For this review, take the finished solid that the model builds, in its own axes (mm). A direction names the side the tool comes from. Give positions to 0.01 mm unless a question says otherwise; leave off trailing zeros. Write each loop counter-clockwise with the first axis right and the second up, starting at its lowest first coordinate (ties: lowest second). Pieces come first, ordered by that corner, then holes.
from build123d import *

# Parameters (mm, degrees)
SKETCH1_W                = 79.7
SKETCH1_H                = 100
SKETCH1_R                = 3.5
SKETCH1_W_2              = 10.2
SKETCH1_H_2              = 10.2
SKETCH1_W_3              = 11
SKETCH1_H_3              = 3
SKETCH1_W_4              = 3
BOSS_EXTRUDE1_DEPTH      = 2
BOSS_EXTRUDE2_DEPTH      = 2
BOSS_EXTRUDE2_DEPTH_BACK = 10
SKETCH1_3_W              = 83.7
SKETCH1_3_H              = 104
SKETCH1_3_W_2            = 79.7
SKETCH1_3_H_2            = 100


with BuildPart() as part:
    # Sketch1 → Boss-Extrude1 (new body)
    with BuildSketch(Plane(origin=(0, 0, 0), x_dir=(1, 0, 0), z_dir=(0, 1, 0))):
        with Locations((-77.999694214, 27.678571429)):
            Rectangle(SKETCH1_W, SKETCH1_H)
        with Locations(Location((-102.849694214, 35.042631833, 0), (0, 0, 270))):
            Circle(SKETCH1_R, mode=Mode.SUBTRACT)
        with Locations(Location((-86.349694214, 35.042631833, 0), (0, 0, 270))):
            Circle(SKETCH1_R, mode=Mode.SUBTRACT)
        with Locations(Location((-69.849694214, 35.042631833, 0), (0, 0, 270))):
            Circle(SKETCH1_R, mode=Mode.SUBTRACT)
        with Locations(Location((-53.349694214, 35.042631833, 0), (0, 0, 270))):
            Circle(SKETCH1_R, mode=Mode.SUBTRACT)
        with Locations(Location((-102.849694214, 50.042631833, 0), (0, 0, 270))):
            Circle(SKETCH1_R, mode=Mode.SUBTRACT)
        with Locations(Location((-86.349694214, 50.042631833, 0), (0, 0, 270))):
            Circle(SKETCH1_R, mode=Mode.SUBTRACT)
        with Locations(Location((-69.849694214, 50.042631833, 0), (0, 0, 270))):
            Circle(SKETCH1_R, mode=Mode.SUBTRACT)
        with Locations(Location((-53.349694214, 50.042631833, 0), (0, 0, 270))):
            Circle(SKETCH1_R, mode=Mode.SUBTRACT)
        with Locations((-86.249694214, -10.078571429)):
            Rectangle(SKETCH1_W_2, SKETCH1_H_2, mode=Mode.SUBTRACT)
        with Locations((-102.749694214, -10.078571429)):
            Rectangle(SKETCH1_W_2, SKETCH1_H_2, mode=Mode.SUBTRACT)
        with Locations((-69.749694214, -10.078571429)):
            Rectangle(SKETCH1_W_2, SKETCH1_H_2, mode=Mode.SUBTRACT)
        with Locations((-53.249694214, -10.078571429)):
            Rectangle(SKETCH1_W_2, SKETCH1_H_2, mode=Mode.SUBTRACT)
        with Locations((-86.249694214, 14.921428571)):
            Rectangle(SKETCH1_W_2, SKETCH1_H_2, mode=Mode.SUBTRACT)
        with Locations((-102.749694214, 14.921428571)):
            Rectangle(SKETCH1_W_2, SKETCH1_H_2, mode=Mode.SUBTRACT)
        with Locations((-69.749694214, 14.921428571)):
            Rectangle(SKETCH1_W_2, SKETCH1_H_2, mode=Mode.SUBTRACT)
        with Locations((-53.249694214, 14.921428571)):
            Rectangle(SKETCH1_W_2, SKETCH1_H_2, mode=Mode.SUBTRACT)
        with Locations((-78.657921682, 69.115214956)):
            Rectangle(SKETCH1_W_3, SKETCH1_H_3, mode=Mode.SUBTRACT)
        with Locations((-112.817389032, 69.702349137)):
            Rectangle(SKETCH1_W_4, SKETCH1_H_2, mode=Mode.SUBTRACT)
        with Locations((-105.072966437, 69.702349137)):
            Rectangle(SKETCH1_W_2, SKETCH1_H_2, mode=Mode.SUBTRACT)
    extrude(amount=BOSS_EXTRUDE1_DEPTH)

    # Sketch1<3> → Boss-Extrude2 (add, two sides: drawn at the far end of the back side and taken through both)
    with BuildSketch(Plane(origin=(0, 0, 0), x_dir=(1, 0, 0), z_dir=(0, 1, 0)).offset(-BOSS_EXTRUDE2_DEPTH_BACK)):
        with Locations((-77.999694214, 27.678571429)):
            Rectangle(SKETCH1_3_W, SKETCH1_3_H)
        with Locations((-77.999694214, 27.678571429)):
            Rectangle(SKETCH1_3_W_2, SKETCH1_3_H_2, mode=Mode.SUBTRACT)
    extrude(amount=BOSS_EXTRUDE2_DEPTH + BOSS_EXTRUDE2_DEPTH_BACK)


solid = part.part
(1) For L1, parallel to Z at x = -53, y = -8.5; L2, parallel to X at y = -0.5, z = -65.5; L3, parallel to Z at x = -81.5, y = 0.75, list the stretches that pass through material, from the lowest coordinate up.
(2) We need section C-C (z = -72). Write out the cut boundary in (x, y), and give its area (3 significant figures).
(3) We need section B-B (y = -1.25). Write out the cut boundary in (x, z).
(4) We need section D-D (x = -92.5). Write out the cut boundary in (y, z), and give its area (3 significant figures).
(5) The part is to be moulded in two halves that separate along X. For faces 3 (the cylindrical face through (-50.98, 0.99, -37.62)), 4 (the flat face through (-36.15, -4, -27)), 5 (the flat face through (-119.85, -4, -27)), 6 (the flat face through (-79, -4, 24.321)), say which applies: +X half, -X half, draft (parallel to the pull), parting line (faces both ways), or undercut.
(6) Tool access review of faces 1 (the flat face through (-79, 0, -28)), 2 (the flat face through (-78, -10, -78)): name each direction out of +Z, -Z, +X, -X, +Y, -Y from which nothing blocks a thin tool from reaching the whole face with its end or side.
(7) Clearance check with a flat-ended pin moving along its axis: pin 1 Ø1.5 at (x, z) = (-49.5, -25) entering from -Y. State where the tip first meets the part, or that it passes through.
(8) We need section A-A (z = 7). Write out the cut boundary in (x, y).
The answers:
1. L1: z = -79.68 to -77.68, 22.32 to 24.32
1. L2: x = -119.85 to -117.85, -38.15 to -36.15
1. L3: z = -79.68 to -70.62, -67.62 to -20.02, -9.82 to 4.98, 15.18 to 24.32
2. outline: (-119.85, -10) - (-117.85, -10) - (-117.85, 0) - (-114.32, 0) - (-114.32, 2) - (-119.85, 2) - close; (-111.32, 0) - (-110.17, 0) - (-110.17, 2) - (-111.32, 2) - close; (-99.97, 0) - (-38.15, 0) - (-38.15, -10) - (-36.15, -10) - (-36.15, 2) - (-99.97, 2) - close
2. area: 181 mm2
3. outline: (-119.85, -79.68) - (-36.15, -79.68) - (-36.15, 24.32) - (-119.85, 24.32) - close; hole (-117.85, -77.68) - (-38.15, -77.68) - (-38.15, 22.32) - (-117.85, 22.32) - close
4. outline: (-10, -79.68) - (2, -79.68) - (2, 24.32) - (-10, 24.32) - (-10, 22.32) - (0, 22.32) - (0, -77.68) - (-10, -77.68) - close
4. area: 248 mm2
5. face 3: undercut
5. face 4: +X half
5. face 5: -X half
5. face 6: draft
6. face 1: -Y
6. face 2: +Z, -Z, +X, -X, -Y
7. pin 1: stops at y = 0
8. outline: (-119.85, -10) - (-117.85, -10) - (-117.85, 0) - (-107.85, 0) - (-107.85, 2) - (-119.85, 2) - close; (-97.65, 0) - (-91.35, 0) - (-91.35, 2) - (-97.65, 2) - close; (-81.15, 0) - (-74.85, 0) - (-74.85, 2) - (-81.15, 2) - close; (-64.65, 0) - (-58.35, 0) - (-58.35, 2) - (-64.65, 2) - close; (-48.15, 0) - (-38.15, 0) - (-38.15, -10) - (-36.15, -10) - (-36.15, 2) - (-48.15, 2) - close
